Can you work these out from the model? Positions are in its coordinate system, mm. A direction names the side the tool comes from. Give positions to 0.01 mm unless a question says otherwise; leave off trailing zeros. Write each loop counter-clockwise with the first axis right and the second up, starting at its lowest first coordinate (ties: lowest second). Pieces come first, ordered by that corner, then holes.
1. On a 3-axis mill with a long thin cutter (end or side, diameter ignored), from which of +Z, -Z, +X, -X, +Y, -Y can I reach the whole of each face in a straight line? I mean faces 4 (the flat face through (-23, 0, 31.866)), 5 (the cylindrical face through (53.84, 27.915, 31.321)). Say none if no direction works.
2. I'm going to push flat-ended pins straight in: pin 1 (17.5 mm diameter, centred on x = -22.3, y = 0, fed in from +Z); pin 2 (4 mm diameter, centred on y = 21, z = 52.5, fed in from +X); pin 3 (1.5 mm diameter, centred on y = 25.5, z = 55, fed in from +X). Where does each tip first touch, or does it pass through?
3. Suppose I cut it at A-A (z = 46). Please give me the cut outline in (x, y).
4. Suppose I cut it at D-D (y = -5). Please give me the cut outline in (x, z).
5. Thinking about a two-plate mould opening in X: for faces 1 (the cylindrical face through (-33.87, -8.87, 47.03)), 2 (the flat face through (-16, -40.647, 30)), 3 (the flat face through (-65.916, -3, 30)), which applies, pulls with the +X half, pulls with the -X half, needs draft (parallel to the pull), parting line crosses it, or undercut?
6. Suppose I cut it at B-B (y = 4). Please give me the cut outline in (x, z), and give its area (3 significant figures).
7. Suppose I cut it at C-C (z = 13). Please give me the cut outline in (x, y), and give its area (3 significant figures).
8. If I drill on probe 1 along Z at (x, y) = (-21.5, 6.5); probe 2 along Y at (x, z) = (-34, 50); probe 3 along X at (y, z) = (7, 50), over which ranges is the centre line in solid material (lowest first)?
```python
from build123d import *

# Parameters (mm, degrees)
F0_W     = 127
F0_H     = 76.2
F1_DEPTH = 61.777094
F2_R     = 25.4
F3_R     = 14.58048
F4_DEPTH = 29.911026


with BuildPart() as f1:
    # F0 (on Top) → F1 (new body)
    with BuildSketch(Plane.XY):
        with Locations((-2.416426, -2.546754)):
            Rectangle(F0_W, F0_H)
    extrude(amount=F1_DEPTH)

    # F2
    f2_edges = [f1.edges().sort_by_distance(p)[0] for p in [
        (61.083574, -40.646754, 30.888547),
        (61.083574, 35.553246, 30.888547),
    ]]
    fillet(f2_edges, radius=F2_R)

    # F3 (on face) → F4 (cut)
    with BuildSketch(Plane.XY.offset(61.777094)):
        with Locations((-22.297775, 0)):
            Circle(F3_R)
    extrude(amount=-F4_DEPTH, mode=Mode.SUBTRACT)


solid = f1.part
```
Checks:
1. face 4: +Z
1. face 5: +Z, -Z, +X, +Y
2. pin 1: stops at z = 31.87
2. pin 2: stops at x = 59.49
2. pin 3: stops at x = 56.47
3. outline: (-65.92, -40.65) - (35.68, -40.65) arc R25.4 ccw to (61.08, -15.25) - (61.08, 10.15) arc R25.4 ccw to (35.68, 35.55) - (-65.92, 35.55) - close; hole circle Ø29.16 at (-22.3, 0)
4. outline: (-65.92, 0) - (61.08, 0) - (61.08, 61.78) - (-8.6, 61.78) - (-8.6, 31.87) - (-35.99, 31.87) - (-35.99, 61.78) - (-65.92, 61.78) - close
5. face 1: undercut
5. face 2: needs draft
5. face 3: pulls with the -X half
6. outline: (-65.92, 0) - (61.08, 0) - (61.08, 61.78) - (-8.28, 61.78) - (-8.28, 31.87) - (-36.32, 31.87) - (-36.32, 61.78) - (-65.92, 61.78) - close
6. area: 7,010 mm2
7. outline: (-65.92, -40.65) - (35.68, -40.65) arc R25.4 ccw to (61.08, -15.25) - (61.08, 10.15) arc R25.4 ccw to (35.68, 35.55) - (-65.92, 35.55) - close
7. area: 9,400 mm2
8. probe 1: z = 0 to 31.87
8. probe 2: y = -40.65 to -8.7, 8.7 to 35.55
8. probe 3: x = -65.92 to -35.09, -9.51 to 61.08
